Here's how the part is built. I have some questions about the finished solid (model axes, mm). Face numbers are marked on the shaded views. Coordinates: 2 decimals unless noted, no trailing zeros. Write each loop counter-clockwise with the first axis right and the second up, starting at its lowest first coordinate (ties: lowest second). Pieces come first, ordered by that corner, then holes.
Item 1: I want a section at D-D (z = -10). Please give me the cut outline in (x, y), and give its area (4 significant figures).
Item 2: I want a section at B-B (y = 0.95). Please give me the cut outline in (x, z), and give its area (3 significant figures).
Item 3: I want a section at A-A (x = -27.15). Please give me the cut outline in (y, z), and give its area (3 significant figures).
Item 4: I want a section at C-C (z = 0). Please give me the cut outline in (x, y), and give its area (3 significant figures).
Item 5: Please list where these lines run through material, in increasing order: line 1 (X direction, y = 0.4, z = 0); line 2 (Z direction, x = 3.5, y = 1.5); line 3 (X direction, y = 0.7, z = 0).
Item 6: I'm going to push flat-ended pins straight in: P1, Ø0.6, axis at y = 1.5, z = -22, coming from the +X side; P2, Ø0.8, axis at x = -28, y = 1, coming from the -Z side; P3, Ø5, axis at x = 12.5, z = -15.5, coming from the +Y side. Where does each tip first touch, or does it pass through?
Item 7: If we mould it in two halves opening along Z, with no side actions, what happens to the marked faces 1 and 2? For each: pulls with the +Z half, pulls with the -Z half, needs draft (parallel to the pull), parting line crosses it, or undercut.
Autodesk Inventor part; units mm, degrees
ref_plane "YZ Plane" through (0, 0, 0) normal (1, 0, 0) x (0, 1, 0)
ref_plane "XZ Plane" through (0, 0, 0) normal (0, 1, 0) x (-1, 0, 0)
ref_plane "XY Plane" through (0, 0, 0) normal (0, 0, 1) x (1, 0, 0)
sketch "Sketch1" plane through (0, 0, 0) normal (0, 1, 0) x (-1, 0, 0)
  line L0 (-28.75, -22.05) -> (28.75, -22.05)
  line L1 (28.75, -22.05) -> (28.75, 22.05)
  line L2 (28.75, 22.05) -> (-28.75, 22.05)
  line L3 (-28.75, 22.05) -> (-28.75, -22.05)
  line L4 (-28.75, -22.05) -> (28.75, 22.05) construction
  line L5 (28.75, -22.05) -> (-28.75, 22.05) construction
  point P0 (0, 0)
  dimension "d2" = 44.1
  dimension "d3" = 57.5
extrude "Extrusion1" add sketch "Sketch1" along normal blind 0.5
sketch "Sketch2" plane through (0, 0.5, 0) normal (0, 1, 0) x (1, 0, 0)
  line L0 (-28.75, 22.05) -> (-28.75, -22.05)
  line L1 (28.75, 22.05) -> (-28.75, 22.05)
  line L2 (-28.75, -22.05) -> (-27.75, -22.05)
  line L3 (-27.75, -22.05) -> (-27.75, 22.05)
  line L4 (-27.75, 22.05) -> (-28.75, 22.05)
  line L5 (-28.75, 22.05) -> (-28.75, -22.05)
  line L6 (28.75, -22.05) -> (27.75, -22.05)
  line L7 (27.75, -22.05) -> (27.75, 22.05)
  line L8 (27.75, 22.05) -> (28.75, 22.05)
  line L9 (28.75, 22.05) -> (28.75, -22.05)
  point P0 (0, 0)
  dimension "d4" = 1
  dimension "d5" = 1
extrude "Extrusion2" add sketch "Sketch2" along normal blind 1.3
sketch "Sketch3" plane through (0, 0, 0) normal (0, -1, 0) x (1, 0, 0)
  line L0 (28.75, 22.05) -> (28.75, -22.05)
  line L1 (-28.75, -22.05) -> (-28.75, 22.05)
  point P0 (0, 0)
  point P1 (-27.15, 0)
  point P2 (27.15, 0)
  dimension "d8" = 1.6
  dimension "d9" = 1.6
hole "Hole1" at (-27.15, 0, 0) at (27.15, 0, 0) direction (0, 1, 0) diameter 2.5 depth 6.3 tip angle 118
sketch "Sketch4" plane through (0, 0.5, 0) normal (0, 1, 0) x (1, 0, 0)
  line L0 (27.75, -22.05) -> (28.75, -22.05)
  line L1 (-27.75, -1.0966) -> (-27.75, -22.05)
  line L2 (27.75, -22.05) -> (-27.75, -22.05)
  line L3 (-27.75, -22.05) -> (-27.75, -21.55)
  line L4 (-27.75, -21.55) -> (27.75, -21.55)
  line L5 (27.75, -21.55) -> (27.75, -22.05)
  line L6 (-27.75, 22.05) -> (27.75, 22.05)
  line L7 (27.75, 22.05) -> (27.75, 21.55)
  line L8 (27.75, 21.55) -> (-27.75, 21.55)
  line L9 (-27.75, 21.55) -> (-27.75, 22.05)
  point P0 (0, 0)
  dimension "d17" = 0.5
  dimension "d18" = 0.5
extrude "Extrusion3" add sketch "Sketch4" along normal blind 1.3
sketch "Sketch5" plane through (0, 1.8, 0) normal (0, 1, 0) x (1, 0, 0)
  line L0 (28.75, -22.05) -> (28.75, 22.05)
  line L1 (28.75, -22.05) -> (18.75, -22.05)
  line L2 (18.75, -22.05) -> (18.75, -12.05)
  line L3 (18.75, -12.05) -> (28.75, -12.05)
  line L4 (28.75, -12.05) -> (28.75, -22.05)
  line L5 (28.75, 22.05) -> (18.75, 22.05)
  line L6 (18.75, 22.05) -> (18.75, 12.05)
  line L7 (18.75, 12.05) -> (28.75, 12.05)
  line L8 (28.75, 12.05) -> (28.75, 22.05)
  line L9 (-28.75, 22.05) -> (-18.75, 22.05)
  line L10 (-18.75, 22.05) -> (-18.75, 12.05)
  line L11 (-18.75, 12.05) -> (-28.75, 12.05)
  line L12 (-28.75, 12.05) -> (-28.75, 22.05)
  line L13 (-28.75, -22.05) -> (-18.75, -22.05)
  line L14 (-18.75, -22.05) -> (-18.75, -12.05)
  line L15 (-18.75, -12.05) -> (-28.75, -12.05)
  line L16 (-28.75, -12.05) -> (-28.75, -22.05)
  point P0 (0, 0)
  dimension "d21" = 10
  dimension "d22" = 10
  dimension "d23" = 10
  dimension "d24" = 10
  dimension "d25" = 10
  dimension "d26" = 10
  dimension "d27" = 10
  dimension "d28" = 10
extrude "Extrusion4" cut sketch "Sketch5" against normal up to surface (1.3 mm away)
equation "\"d5\" = d4"
equation "\"d18\" = d17"
equation "\"d23\" = d21"
equation "\"d24\" = d21"
equation "\"d25\" = d21"
equation "\"d26\" = d22"
equation "\"d27\" = d22"
equation "\"d28\" = d22"
properties part number "Digital Module Cover V2 - Slim"
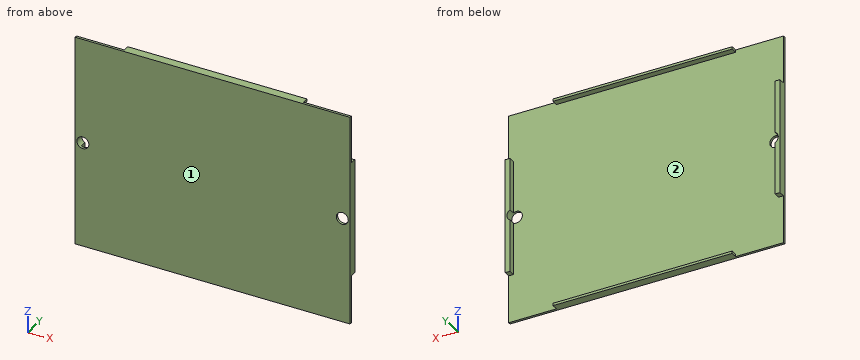
Answer:
1. outline: (-28.75, 0) - (28.75, 0) - (28.75, 1.8) - (27.75, 1.8) - (27.75, 0.5) - (-27.75, 0.5) - (-27.75, 1.8) - (-28.75, 1.8) - close
1. area: 31.35 mm2
2. outline: (-28.75, -12.05) - (-27.75, -12.05) - (-27.75, -1.1) arc R1.25 cw to (-27.75, 1.1) - (-27.75, 12.05) - (-28.75, 12.05) - close; (-18.75, -22.05) - (18.75, -22.05) - (18.75, -21.55) - (-18.75, -21.55) - close; (-18.75, 21.55) - (18.75, 21.55) - (18.75, 22.05) - (-18.75, 22.05) - close; (27.75, -12.05) - (28.75, -12.05) - (28.75, 12.05) - (27.75, 12.05) - (27.75, 1.1) arc R1.25 cw to (27.75, -1.1) - close
2. area: 83.7 mm2
3. outline: (0, -22.05) - (0.5, -22.05) - (0.5, -1.25) - (0, -1.25) - close; (0, 1.25) - (0.5, 1.25) - (0.5, 22.05) - (0, 22.05) - close
3. area: 20.8 mm2
4. outline: (-28.75, 0) - (-28.4, 0) - (-28.4, 1.8) - (-28.75, 1.8) - close; (-25.9, 0) - (25.9, 0) - (25.9, 0.5) - (-25.9, 0.5) - close; (28.4, 0) - (28.75, 0) - (28.75, 1.8) - (28.4, 1.8) - close
4. area: 27.2 mm2
5. line 1: x = -28.75 to -28.4, -25.9 to 25.9, 28.4 to 28.75
5. line 2: z = -22.05 to -21.55, 21.55 to 22.05
5. line 3: x = -28.75 to -28.4, 28.4 to 28.75
6. P1: stops at x = 18.75
6. P2: stops at z = -12.05
6. P3: stops at y = 0.5
7. face 1: needs draft
7. face 2: undercut
